CAD build for the part. Positions are in the model's coordinates, mm. Face numbers are marked on the shaded views. A direction names the side the tool comes from. Round coordinates to 2 decimals unless told otherwise and drop trailing zeros. Loops run counter-clockwise (first coordinate to the right, second up) from the corner with the lowest first, then second, coordinate; pieces in that order, holes last.
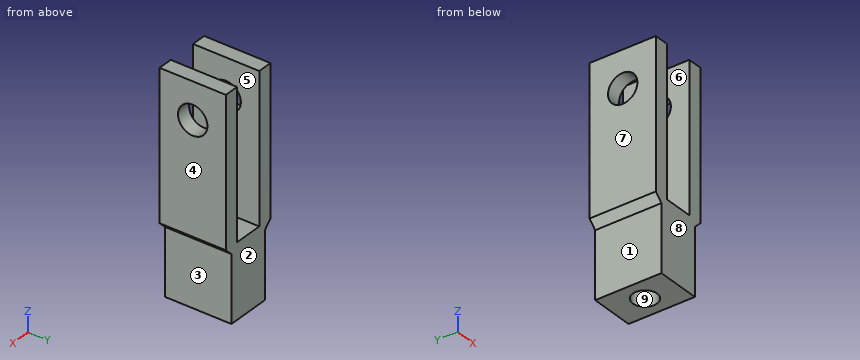
from build123d import *

# Parameters (mm, degrees)
SKETCH1_W             = 6
SKETCH1_H             = 9
BOSS_EXTRUDE1_DEPTH   = 10
M4_TAPPED_HOLE2_D     = 3.3
M4_TAPPED_HOLE2_DEPTH = 8
M4_TAPPED_HOLE2_TIP   = 0.991420021
SKETCH11_W            = 2
SKETCH11_H            = 9
BOSS_EXTRUDE5_DEPTH   = 20
SKETCH12_R            = 2
CUT_EXTRUDE1_DEPTH    = 2
CHAMFER1_SIZE         = 1
CHAMFER2_SIZE         = 1


with BuildPart() as part:
    # Sketch1 → Boss-Extrude1 (new body)
    with BuildSketch(Plane.XY):
        Rectangle(SKETCH1_W, SKETCH1_H)
    extrude(amount=BOSS_EXTRUDE1_DEPTH)

    # M4 Tapped Hole2
    with Locations(Plane(origin=(0, 0, 0), x_dir=(-1, 0, 0), z_dir=(0, 0, -1))):
        with Locations((0, 0)):
            Hole(M4_TAPPED_HOLE2_D / 2, depth=M4_TAPPED_HOLE2_DEPTH)
            with Locations((0, 0, -(M4_TAPPED_HOLE2_DEPTH + M4_TAPPED_HOLE2_TIP / 2))):  # 118° drill point
                Cone(0, M4_TAPPED_HOLE2_D / 2, M4_TAPPED_HOLE2_TIP, mode=Mode.SUBTRACT)

    # Sketch11 → Boss-Extrude5 (add)
    with BuildSketch(Plane.XY.offset(10)):
        with Locations((3, 0)):
            Rectangle(SKETCH11_W, SKETCH11_H)
    boss_extrude5 = extrude(amount=BOSS_EXTRUDE5_DEPTH)

    # Sketch12 → Cut-Extrude1 (cut)
    with BuildSketch(Plane(origin=(4, 0, 0), x_dir=(0, 0, -1), z_dir=(1, 0, 0))):
        with Locations(Location((-25, 0, 0), (0, 0, 90))):
            Circle(SKETCH12_R)
    cut_extrude1 = extrude(amount=-CUT_EXTRUDE1_DEPTH, mode=Mode.SUBTRACT)

    # Mirror1: Boss-Extrude5, Cut-Extrude1 across plane
    add(boss_extrude5.mirror(Plane(origin=(0, 0, 0), x_dir=(0, 0, 1), z_dir=(1, 0, 0))))
    add(cut_extrude1.mirror(Plane(origin=(0, 0, 0), x_dir=(0, 0, 1), z_dir=(1, 0, 0))), mode=Mode.SUBTRACT)

    # Chamfer1
    chamfer1_edges = [part.edges().sort_by_distance(p)[0] for p in [
        (3, 0, 10),
    ]]
    chamfer(chamfer1_edges, length=CHAMFER1_SIZE - 0.0001)  # a hair under: the kernel refuses the full size

    # Chamfer2
    chamfer2_edges = [part.edges().sort_by_distance(p)[0] for p in [
        (-3, 0, 10),
    ]]
    chamfer(chamfer2_edges, length=CHAMFER2_SIZE - 0.0001)  # a hair under: the kernel refuses the full size


solid = part.part
Item 1: Cut at C-C (x = 3.5). List the corners of the cut face in (y, z).
Verdict:
outline: (-4.5, 9.5) - (4.5, 9.5) - (4.5, 30) - (-4.5, 30) - close; hole circle Ø4 at (0, 25)
Item 2: Mould opens along X. For the marked faces 6, 7, 8 and 9 say: released by +X, released by -X, zero draft, split by the parting line, or undercut.
Verdict:
face 6: undercut
face 7: released by -X
face 8: zero draft
face 9: undercut
Item 3: Wall check: L1, parallel to X at y = 3.5, z = 25.5; L2, parallel to Y at x = 0, z = 4.5; L3, parallel to Z at x = -2.9, y = 0. Give the ranges that are in metal, low to high.
Verdict:
L1: x = -4 to -2, 2 to 4
L2: y = -4.5 to -1.65, 1.65 to 4.5
L3: z = 0 to 23, 27 to 30
Item 4: Cut at A-A (z = 22.25). List the corners of the cut face in (x, y), plus the area to 3 significant figures.
Verdict:
outline: (-4, -4.5) - (-2, -4.5) - (-2, 4.5) - (-4, 4.5) - close; (2, -4.5) - (4, -4.5) - (4, 4.5) - (2, 4.5) - close
area: 36.0 mm2
Item 5: 3-axis set-ups, long thin cutter, end or side, ignore diameter. For the marked faces 1, 2, 3, 4 and 5: which of +Z, -Z, +X, -X, +Y, -Y reach the whole face in a straight line?
Verdict:
face 1: -Z, -X, +Y, -Y
face 2: +Z, -Z, +X, -X, +Y
face 3: -Z, +X, +Y, -Y
face 4: +Z, -Z, +X, +Y, -Y
face 5: +Z, +Y, -Y
Item 6: Flat gauge pins, fed straight in: P1, Ø2.5, axis at y = -1, z = 2.5, coming from the +X side; P2, Ø4.5, axis at y = -0.5, z = 6, coming from the -X side; P3, Ø3, axis at x = 0, y = 0, coming from the +Z side. Where does each tip first touch, or does it go through?
Verdict:
P1: stops at x = 3
P2: stops at x = -3
P3: stops at z = 10
